For this review, take the finished solid that the model builds, in its own axes (mm). A direction names the side the tool comes from. Coordinates: 2 decimals unless noted, no trailing zeros. Loops run counter-clockwise (first coordinate to the right, second up) from the corner with the lowest first, then second, coordinate; pieces in that order, holes last. Notation, with made-up numbers: M 83.5,-12.75 L 113.5,-12.75 A20 cw 113.5,5.25 Z; hole C 40.25,-21.75 d1. An arc over 180 degrees is marked long. Write item = value, one per line.
from build123d import *

# Parameters (mm, degrees)
SKETCH1_R           = 30.25
SKETCH1_R_2         = 25.25
EXTRUDE_THIN1_DEPTH = 2
SKETCH2_R           = 1.65
CUT_EXTRUDE3_DEPTH  = 10
BOSS_EXTRUDE1_DEPTH = 2


with BuildPart() as part:
    # Sketch1 → Extrude-Thin1 (new body)
    with BuildSketch(Plane(origin=(0, 0, 0), x_dir=(1, 0, 0), z_dir=(0, 1, 0))):
        Circle(SKETCH1_R)
        Circle(SKETCH1_R_2, mode=Mode.SUBTRACT)
    extrude(amount=-EXTRUDE_THIN1_DEPTH)

    # Sketch2 → Cut-Extrude3 (cut)
    with BuildSketch(Plane(origin=(0, 0, 0), x_dir=(1, 0, 0), z_dir=(0, 1, 0))):
        with Locations((0, 27.5)):
            Circle(SKETCH2_R)
        with Locations((23.815698604, -13.75)):
            Circle(SKETCH2_R)
        with Locations((-23.815698604, -13.75)):
            Circle(SKETCH2_R)
    extrude(amount=-CUT_EXTRUDE3_DEPTH, mode=Mode.SUBTRACT)

    # Sketch5 → Boss-Extrude1 (add)
    with BuildSketch(Plane.XZ.offset(2)):
        with BuildLine():
            Line((0, 50.25), (0, 30.25))
            ThreePointArc((0, 30.25), (3.948417315, 29.991207057), (7.829276114, 29.219256245))
            Line((7.829276114, 29.219256245), (13.005657016, 48.537772771))
            ThreePointArc((13.005657016, 48.537772771), (6.558941159, 49.820104284), (0, 50.25))
        make_face()
        with BuildLine():
            Line((32.300077387, 38.493733267), (19.444325193, 23.172844404))
            ThreePointArc((19.444325193, 23.172844404), (22.302639439, 20.43660378), (24.77934934, 17.3506872))
            Line((24.77934934, 17.3506872), (41.162390226, 28.822215927))
            ThreePointArc((41.162390226, 28.822215927), (37.048186175, 33.948407933), (32.300077387, 38.493733267))
        make_face()
        with BuildLine():
            Line((49.486589589, 8.725820928), (29.790434529, 5.252857374))
            ThreePointArc((29.790434529, 5.252857374), (30.221208703, 1.319486468), (30.134889617, -2.636461218))
            Line((30.134889617, -2.636461218), (50.058783579, -4.379576073))
            ThreePointArc((50.058783579, -4.379576073), (50.202173134, 2.191874215), (49.486589589, 8.725820928))
        make_face()
        with BuildLine():
            Line((43.51777654, -25.125), (26.197268464, -15.125))
            ThreePointArc((26.197268464, -15.125), (23.998938544, -18.415033228), (21.389980131, -21.389980131))
            Line((21.389980131, -21.389980131), (35.532115755, -35.532115755))
            ThreePointArc((35.532115755, -35.532115755), (39.86600535, -30.590261808), (43.51777654, -25.125))
        make_face()
        with BuildLine():
            Line((17.186512202, -47.219554194), (10.346109336, -28.425701779))
            ThreePointArc((10.346109336, -28.425701779), (6.547298322, -29.532954215), (2.636461218, -30.134889617))
            Line((2.636461218, -30.134889617), (4.379576073, -50.058783579))
            ThreePointArc((4.379576073, -50.058783579), (10.8760906, -49.058874358), (17.186512202, -47.219554194))
        make_face()
        with BuildLine():
            Line((-17.186512202, -47.219554194), (-10.346109336, -28.425701779))
            ThreePointArc((-10.346109336, -28.425701779), (-13.96789555, -26.832077704), (-17.3506872, -24.77934934))
            Line((-17.3506872, -24.77934934), (-28.822215927, -41.162390226))
            ThreePointArc((-28.822215927, -41.162390226), (-23.202867815, -44.572294367), (-17.186512202, -47.219554194))
        make_face()
        with BuildLine():
            Line((-43.51777654, -25.125), (-26.197268464, -15.125))
            ThreePointArc((-26.197268464, -15.125), (-27.947355858, -11.576173829), (-29.219256245, -7.829276114))
            Line((-29.219256245, -7.829276114), (-48.537772771, -13.005657016))
            ThreePointArc((-48.537772771, -13.005657016), (-46.424946509, -19.229842476), (-43.51777654, -25.125))
        make_face()
        with BuildLine():
            Line((-49.486589589, 8.725820928), (-29.790434529, 5.252857374))
            ThreePointArc((-29.790434529, 5.252857374), (-28.84993776, 9.096350435), (-27.415810558, 12.784202418))
            Line((-27.415810558, 12.784202418), (-45.541966299, 21.236567652))
            ThreePointArc((-45.541966299, 21.236567652), (-47.924276775, 15.110466425), (-49.486589589, 8.725820928))
        make_face()
        with BuildLine():
            Line((-32.300077387, 38.493733267), (-19.444325193, 23.172844404))
            ThreePointArc((-19.444325193, 23.172844404), (-16.253313152, 25.512591236), (-12.784202418, 27.415810558))
            Line((-12.784202418, 27.415810558), (-21.236567652, 45.541966299))
            ThreePointArc((-21.236567652, 45.541966299), (-26.999305319, 42.380420152), (-32.300077387, 38.493733267))
        make_face()
    extrude(amount=-BOSS_EXTRUDE1_DEPTH)


solid = part.part
Q1. For pin 1 Ø5.5 at (x, z) = (23.82, 13.75) entering from -Y; pin 2 Ø1 at (y, z) = (-1, 40) entering from -X, all flat-tipped, find the tip position at first contact; note any pin that passes through.
Solved:
pin_1 = -2
pin_2 = -31.06
Q2. For line 1 along X through (y, z) = (-0.65, -27.5); line 2 along Z through (x, y) = (-22, -1.2); line 3 along X through (y, z) = (-1.55, 13.5), list the stretches that pass through material, from the lowest coordinate up.
Solved:
line_1 = -19.26 to -1.65, 1.65 to 12.6, 27.5 to 42.06
line_2 = -45.18 to -31.42, -20.76 to -12.39, 12.39 to 20.76, 26.22 to 45.18
line_3 = -48.4 to -28.95, -27.07 to -25.45, -22.18 to -21.34, 21.34 to 22.18, 25.45 to 27.07
Q3. Machinability: for faces 1 (the face through (-13.814, -1.014, -37.954)), 2 (the face through (-22.24, -0.986, -20.505)), 3 (the face through (32.86, -1.01, 23.01)), 4 (the face through (-25.96, -1.01, 30.94)), which of the approach directions +Z, -Z, +X, -X, +Y, -Y give a long, thin tool a straight path to every point of the face, cutting with its end or side? Answer none if there is none.
Solved:
face_1 = -Z, +Y, -Y
face_2 = +Y, -Y
face_3 = +X, +Y, -Y
face_4 = -X, +Y, -Y
Q4. Add section B-B (x = -39). Write out the cut boundary in (y, z), and give its area (3 significant figures).
Solved:
outline = M -2,-22.52 L 0,-22.52 L 0,-10.45 L -2,-10.45 Z; M -2,6.88 L 0,6.88 L 0,18.19 L -2,18.19 Z
area = 46.8 mm²
Q5. Add section A-A (z = 0). Write out the cut boundary in (x, y).
Solved:
outline = M -30.25,-2 L -25.25,-2 L -25.25,0 L -30.25,0 Z; M 25.25,-2 L 50.25,-2 L 50.25,0 L 25.25,0 Z
Q6. Add section C-C (y = -0.3). State how many separate pieces and enclosed holes the cut face has, and give its area (3 significant figures).
Solved:
separate_pieces = 1
enclosed_holes = 4
area = 2,740 mm²
